```python
from build123d import *

# Parameters (mm, degrees)
BOSS_EXTRUDE1_DEPTH = 5
SKETCH2_R           = 1
CUT_EXTRUDE2_DEPTH  = 5


with BuildPart() as part:
    # Sketch1 → Boss-Extrude1 (new body)
    with BuildSketch(Plane(origin=(0, 0, 0), x_dir=(0, 1, 0), z_dir=(0, 0, 1))):
        with BuildLine():
            ThreePointArc((0, 0), (12.744177426, 14.83676339), (32.3, 14.5))
            ThreePointArc((32.3, 14.5), (42.433307292, 26.572812771), (58, 24.1))
            ThreePointArc((58, 24.1), (39.71268336, 40.332103653), (16, 46.3))
            ThreePointArc((16, 46.3), (20.191750993, 33.797330101), (7.055281526, 34.946547632))
            ThreePointArc((7.055281526, 34.946547632), (5.079702, 39.861691185), (4.230496454, 45.090496071))
            ThreePointArc((4.230496454, 45.090496071), (0, 41.9), (-4.230496454, 45.090496071))
            ThreePointArc((-4.230496454, 45.090496071), (-5.079702, 39.861691185), (-7.055281526, 34.946547632))
            ThreePointArc((-7.055281526, 34.946547632), (-20.191750993, 33.797330101), (-16, 46.3))
            ThreePointArc((-16, 46.3), (-39.71268336, 40.332103653), (-58, 24.1))
            ThreePointArc((-58, 24.1), (-42.433307292, 26.572812771), (-32.3, 14.5))
            ThreePointArc((-32.3, 14.5), (-12.744177426, 14.83676339), (0, 0))
        make_face()
    extrude(amount=BOSS_EXTRUDE1_DEPTH)

    # Sketch2 → Cut-Extrude2 (cut)
    with BuildSketch(Plane.XY.offset(5)):
        with Locations((-40, 0)):
            Circle(SKETCH2_R)
    extrude(amount=-CUT_EXTRUDE2_DEPTH, mode=Mode.SUBTRACT)


solid = part.part
```
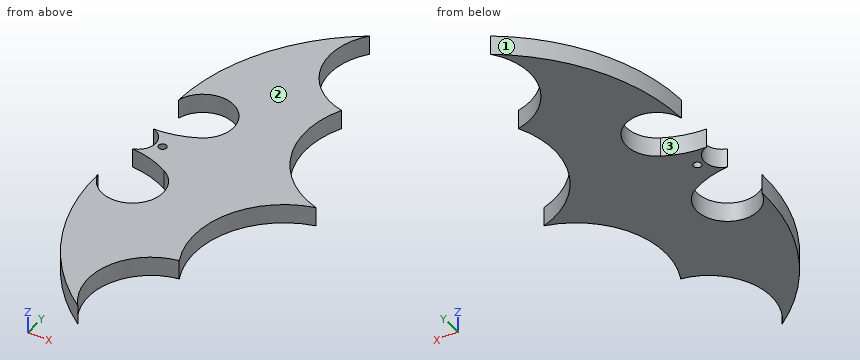
Could you check a few things on this model? Use its own coordinates, in mm. Face numbers are marked on the shaded views. Coordinates: 2 decimals unless noted, no trailing zeros. Loops run counter-clockwise (first coordinate to the right, second up) from the corner with the lowest first, then second, coordinate; pieces in that order, holes last. Notation, with made-up numbers: M 3.25,69 L 42.25,69 A14 ccw 42.25,96 Z; hole C 48.25,16 d9. An arc over 180 degrees is marked long. Put each result on its own line as item: value. Start each with the question number.
(1) I need wall thicknesses on line 1 (Y direction, x = -40, z = 2.5); line 2 (Y direction, x = -37, z = 4.05); line 3 (X direction, y = 18, z = 4.4). Which ranges of each line are inside material? Lowest first, please. Write a range as from..to.
(2) Thinking about a two-plate mould opening in Y: for the marked faces 1, 2 and 3, which applies, pulls with the +Y half, pulls with the -Y half, needs draft (parallel to the pull), parting line crosses it, or undercut?
(3) Suppose I cut it at A-A on z = 3.55. Please give me the cut outline in (x, y) (1 decimal), then the cut area to 3 significant figures.
(4) Will these pins go through, and if not, where does the flat tip stop? P1, Ø3, axis at y = -24.5, z = 1.5, coming from the -X side; P2, Ø18, axis at x = -38.68, y = 14, coming from the -Z side.
(5) Suppose I cut it at D-D on x = -9. Please give me the cut outline in (y, z).
(6) Suppose I cut it at C-C on y = -12.5. Please give me the cut outline in (x, z).
(7) Suppose I cut it at B-B on x = -38. Please give me the cut outline in (y, z).
Solutions:
1. line 1: y = -40.33..-21.77, -5.04..-1, 1..5.04, 21.77..40.33
1. line 2: y = -45.17..-21.7, -6.08..6.08, 21.7..45.17
1. line 3: x = -46.25..-45.47, -31.88..-16.47
2. face 1: pulls with the +Y half
2. face 2: needs draft
2. face 3: undercut
3. outline: M -46.3,-16 A51.5 ccw -24.1,-58 A16 cw -14.5,-32.3 A23 cw 0,0 A23 cw -14.5,32.3 A16 cw -24.1,58 A51.5 ccw -46.3,16 A7.9 cw long -34.9,7.1 A24 cw -45.1,4.2 A4.4 cw -45.1,-4.2 A24 cw -34.9,-7.1 A7.9 cw long Z; hole C -40,0 d2
3. area: 2,170 mm2
4. P1: stops at x = -45.77
4. P2: stops at z = 0
5. outline: M -4.85,0 L 4.85,0 L 4.85,5 L -4.85,5 Z
6. outline: M -30.94,0 L -14.73,0 L -14.73,5 L -30.94,5 Z
7. outline: M -43.68,0 L -21.85,0 L -21.85,5 L -43.68,5 Z; M -5.68,0 L 5.68,0 L 5.68,5 L -5.68,5 Z; M 21.85,0 L 43.68,0 L 43.68,5 L 21.85,5 Z
